Check sheet for the modelled part. Datum: model origin and axes. Units: mm. Round coordinates to 2 decimals unless told otherwise and drop trailing zeros. Write each loop counter-clockwise with the first axis right and the second up, starting at its lowest first coordinate (ties: lowest second). Pieces come first, ordered by that corner, then holes. Notation, with made-up numbers: (10.5, 37) -> (31.5, 37) arc R35 ccw to (31.5, 72) -> close; hole circle Ø1 at (10.25, 61.5). An arc over 180 degrees is marked (long way). One line per item, written item: value.
from build123d import *

# Parameters (mm, degrees)
SKETCH1_W           = 250
SKETCH1_H           = 45
BOSS_EXTRUDE1_DEPTH = 3.175
SKETCH4_R           = 3
SKETCH4_R_2         = 1.75
CUT_EXTRUDE1_DEPTH  = 227.144490592
SKETCH5_R           = 4.25
CUT_EXTRUDE2_DEPTH  = 227.144490592
SKETCH6_R           = 11.5
SKETCH6_R_2         = 1.5
CUT_EXTRUDE3_DEPTH  = 227.144490592
SKETCH10_R          = 1.75
CUT_EXTRUDE4_DEPTH  = 227.144490592
FILLET1_R           = 7
SKETCH11_R          = 2.5
CUT_EXTRUDE5_DEPTH  = 227.144490592
CUT_EXTRUDE6_DEPTH  = 227.144490592


with BuildPart() as part:
    # Sketch1 → Boss-Extrude1 (new body)
    with BuildSketch(Plane(origin=(0, 0, 0), x_dir=(1, 0, 0), z_dir=(0, 1, 0))):
        with Locations((100, 0)):
            Rectangle(SKETCH1_W, SKETCH1_H)
    extrude(amount=BOSS_EXTRUDE1_DEPTH)

    # Sketch4 → Cut-Extrude1 (cut, through all)
    with BuildSketch(Plane(origin=(0, 3.175, 0), x_dir=(1, 0, 0), z_dir=(0, 1, 0))):
        with Locations(Location((200, 0, 0), (0, 0, 270))):
            Circle(SKETCH4_R)
        with Locations(Location((186, 9, 0), (0, 0, 270))):
            Circle(SKETCH4_R_2)
        with Locations(Location((214, 9, 0), (0, 0, 90))):
            Circle(SKETCH4_R_2)
        with Locations(Location((214, -9, 0), (0, 0, 270))):
            Circle(SKETCH4_R_2)
        with Locations(Location((186, -9, 0), (0, 0, 90))):
            Circle(SKETCH4_R_2)
    extrude(amount=-CUT_EXTRUDE1_DEPTH, mode=Mode.SUBTRACT)

    # Sketch5 → Cut-Extrude2 (cut, through all)
    with BuildSketch(Plane(origin=(0, 3.175, 0), x_dir=(1, 0, 0), z_dir=(0, 1, 0))):
        with Locations(Location((0, 0, 0), (0, 0, 270))):
            Circle(SKETCH5_R)
    extrude(amount=-CUT_EXTRUDE2_DEPTH, mode=Mode.SUBTRACT)

    # Sketch6 → Cut-Extrude3 (cut, through all)
    with BuildSketch(Plane(origin=(0, 3.175, 0), x_dir=(1, 0, 0), z_dir=(0, 1, 0))):
        with Locations(Location((45, 0, 0), (0, 0, 270))):
            Circle(SKETCH6_R)
        with Locations(Location((29.5, 15.5, 0), (0, 0, 270))):
            Circle(SKETCH6_R_2)
        with Locations(Location((60.5, 15.5, 0), (0, 0, 90))):
            Circle(SKETCH6_R_2)
        with Locations(Location((60.5, -15.5, 0), (0, 0, 270))):
            Circle(SKETCH6_R_2)
        with Locations(Location((29.5, -15.5, 0), (0, 0, 90))):
            Circle(SKETCH6_R_2)
    extrude(amount=-CUT_EXTRUDE3_DEPTH, mode=Mode.SUBTRACT)

    # Sketch10 → Cut-Extrude4 (cut, through all)
    with BuildSketch(Plane(origin=(0, 3.175, 0), x_dir=(1, 0, 0), z_dir=(0, 1, 0))):
        with Locations(Location((80.5, -17.5, 0), (0, 0, 270))):
            Circle(SKETCH10_R)
        with Locations(Location((123.25, -17.5, 0), (0, 0, 270))):
            Circle(SKETCH10_R)
        with Locations(Location((166, -17.5, 0), (0, 0, 270))):
            Circle(SKETCH10_R)
        with Locations(Location((166, 17.5, 0), (0, 0, 90))):
            Circle(SKETCH10_R)
        with Locations(Location((80.5, 17.5, 0), (0, 0, 90))):
            Circle(SKETCH10_R)
        with Locations(Location((123.25, 17.5, 0), (0, 0, 90))):
            Circle(SKETCH10_R)
    extrude(amount=-CUT_EXTRUDE4_DEPTH, mode=Mode.SUBTRACT)

    # Fillet1
    fillet1_edges = [part.edges().sort_by_distance(p)[0] for p in [
        (-25, 1.5875, -22.5),
        (225, 1.5875, -22.5),
        (225, 1.5875, 22.5),
        (-25, 1.5875, 22.5),
    ]]
    fillet(fillet1_edges, radius=FILLET1_R)

    # Sketch11 → Cut-Extrude5 (cut, through all)
    with BuildSketch(Plane(origin=(0, 3.175, 0), x_dir=(1, 0, 0), z_dir=(0, 1, 0))):
        with Locations(Location((0, 17.5, 0), (0, 0, 270))):
            Circle(SKETCH11_R)
        with Locations(Location((17.5, 0, 0), (0, 0, 270))):
            Circle(SKETCH11_R)
        with Locations(Location((0, -17.5, 0), (0, 0, 270))):
            Circle(SKETCH11_R)
        with Locations(Location((-17.5, 0, 0), (0, 0, 270))):
            Circle(SKETCH11_R)
    extrude(amount=-CUT_EXTRUDE5_DEPTH, mode=Mode.SUBTRACT)

    # Sketch12 → Cut-Extrude6 (cut, through all)
    with BuildSketch(Plane(origin=(0, 3.175, 0), x_dir=(1, 0, 0), z_dir=(0, 1, 0))):
        with BuildLine():
            Line((23, 17.1), (75, 17.1))
            ThreePointArc((75, 17.1), (76.060660172, 16.660660172), (76.5, 15.6))
            Line((76.5, 15.6), (76.5, 15.4))
            ThreePointArc((76.5, 15.4), (76.060660172, 14.339339828), (75, 13.9))
            Line((75, 13.9), (23, 13.9))
            ThreePointArc((23, 13.9), (21.939339828, 14.339339828), (21.5, 15.4))
            Line((21.5, 15.4), (21.5, 15.6))
            ThreePointArc((21.5, 15.6), (21.939339828, 16.660660172), (23, 17.1))
        make_face()
        with BuildLine():
            Line((76.5, -15.6), (76.5, -15.4))
            ThreePointArc((76.5, -15.4), (76.060660172, -14.339339828), (75, -13.9))
            Line((75, -13.9), (23, -13.9))
            ThreePointArc((23, -13.9), (21.939339828, -14.339339828), (21.5, -15.4))
            Line((21.5, -15.4), (21.5, -15.6))
            ThreePointArc((21.5, -15.6), (21.939339828, -16.660660172), (23, -17.1))
            Line((23, -17.1), (75, -17.1))
            ThreePointArc((75, -17.1), (76.060660172, -16.660660172), (76.5, -15.6))
        make_face()
        with BuildLine():
            Line((36.75, 11.5), (61.25, 11.5))
            ThreePointArc((61.25, 11.5), (69.204951288, 8.204951288), (72.5, 0.25))
            Line((72.5, 0.25), (72.5, -0.25))
            ThreePointArc((72.5, -0.25), (69.204951288, -8.204951288), (61.25, -11.5))
            Line((61.25, -11.5), (36.75, -11.5))
            ThreePointArc((36.75, -11.5), (28.795048712, -8.204951288), (25.5, -0.25))
            Line((25.5, -0.25), (25.5, 0.25))
            ThreePointArc((25.5, 0.25), (28.795048712, 8.204951288), (36.75, 11.5))
        make_face()
    extrude(amount=-CUT_EXTRUDE6_DEPTH, mode=Mode.SUBTRACT)


solid = part.part
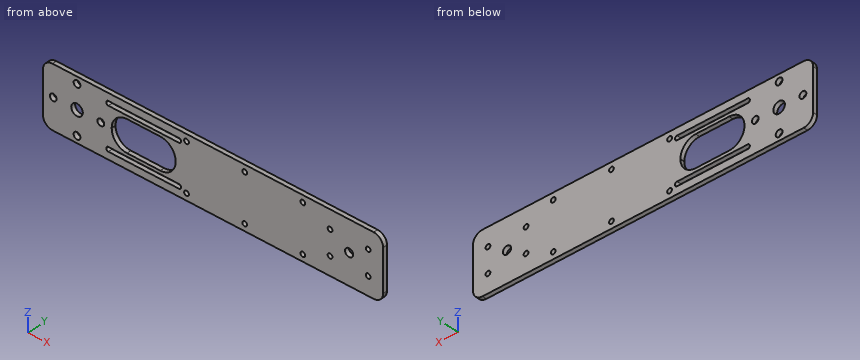
Item 1: Material ranges on line 1 along Z through (x, y) = (186, 2.05); line 2 along X through (y, z) = (1.6, 0.5); line 3 along Z through (x, y) = (166, 1.9), recorded low to high.
Result set:
line 1: -22.5 to -10.75, -7.25 to 7.25, 10.75 to 22.5
line 2: -25 to -19.95, -15.05 to -4.22, 4.22 to 15.05, 19.95 to 25.5, 72.5 to 197.04, 202.96 to 225
line 3: -22.5 to -19.25, -15.75 to 15.75, 19.25 to 22.5
Item 2: Sectioned sample at A-A (x = 42). Enter the section's corners in (y, z) (3 decimals), then the cut area to 3 significant figures.
Result set:
outline: (0, -22.5) -> (3.175, -22.5) -> (3.175, -17.1) -> (0, -17.1) -> close; (0, -13.9) -> (3.175, -13.9) -> (3.175, -11.5) -> (0, -11.5) -> close; (0, 11.5) -> (3.175, 11.5) -> (3.175, 13.9) -> (0, 13.9) -> close; (0, 17.1) -> (3.175, 17.1) -> (3.175, 22.5) -> (0, 22.5) -> close
area: 49.5 mm^2
Item 3: Sectioned sample at B-B (y = 1.45). State how many separate pieces and enclosed holes the cut face has, then the cut area to 3 significant figures.
Result set:
separate pieces: 1
enclosed holes: 19
area: 9,630 mm^2
Item 4: Sectioned sample at C-C (x = 0). Enter the section's corners in (y, z) (3 decimals).
Result set:
outline: (0, -22.5) -> (3.175, -22.5) -> (3.175, -20) -> (0, -20) -> close; (0, -15) -> (3.175, -15) -> (3.175, -4.25) -> (0, -4.25) -> close; (0, 4.25) -> (3.175, 4.25) -> (3.175, 15) -> (0, 15) -> close; (0, 20) -> (3.175, 20) -> (3.175, 22.5) -> (0, 22.5) -> close
